from build123d import *

# Parameters (mm, degrees)
SKETCH1_W                      = 20
SKETCH1_H                      = 16
BOSS_EXTRUDE1_DEPTH            = 11.5
CUT_EXTRUDE1_DEPTH             = 17
SKETCH3_W                      = 3
SKETCH3_H                      = 16
SKETCH4_W                      = 1.5
SKETCH4_H                      = 7
F_6_0_6_DIAMETER_HOLE1_D       = 6
F_6_0_6_DIAMETER_HOLE1_DEPTH   = 11.5
F_3_0_3_DIAMETER_HOLE2_D       = 3
F_3_0_3_DIAMETER_HOLE2_DEPTH   = 3.5
F_3_0_3_DIAMETER_HOLE3_D       = 3
F_3_0_3_DIAMETER_HOLE3_DEPTH   = 3.5
F_1_5_1_5_DIAMETER_HOLE1_D     = 1.5
F_1_5_1_5_DIAMETER_HOLE1_DEPTH = 4.5
CHAMFER1_SIZE                  = 0.25


with BuildPart() as part:
    # Sketch1 → Boss-Extrude1 (new body)
    with BuildSketch(Plane.XZ):
        Rectangle(SKETCH1_W, SKETCH1_H)
    extrude(amount=-BOSS_EXTRUDE1_DEPTH)

    # Sketch2 → Cut-Extrude1 (cut, through all)
    with BuildSketch(Plane(origin=(0, 0, -8), x_dir=(-1, 0, 0), z_dir=(0, 0, -1))):
        with BuildLine():
            Line((10, 3.5), (10, 4.5))
            Line((10, 4.5), (4.458039892, 4.5))
            ThreePointArc((4.458039892, 4.5), (4.5, 4), (4.458039892, 3.5))
            Line((4.458039892, 3.5), (10, 3.5))
        make_face()
    extrude(amount=-CUT_EXTRUDE1_DEPTH, mode=Mode.SUBTRACT)

    # Sketch3 → Cut-Revolve1 (revolve, cut)
    with BuildSketch(Plane(origin=(0, 4, 0), x_dir=(1, 0, 0), z_dir=(0, 1, 0))):
        Rectangle(SKETCH3_W, SKETCH3_H)
    revolve(axis=Axis((-1.5, 4, -8), (0, 0, 1)), mode=Mode.SUBTRACT)

    # Sketch4 → Ø3.0 (3) Diameter Hole1 (revolve, cut)
    with BuildSketch(Plane(origin=(-7.5, 4.5, 0), x_dir=(0, 0, -1), z_dir=(1, 0, 0))):
        with Locations((0.75, 3.5)):
            Rectangle(SKETCH4_W, SKETCH4_H)
    revolve(axis=Axis((-7.5, -1.85, 0), (0, 1, 0)), mode=Mode.SUBTRACT)

    # Ø6.0 (6) Diameter Hole1
    with Locations(Plane(origin=(0, 0, 0), x_dir=(-1, 0, 0), z_dir=(0, -1, 0))):
        with Locations((-5.5, 0)):
            Hole(F_6_0_6_DIAMETER_HOLE1_D / 2, depth=F_6_0_6_DIAMETER_HOLE1_DEPTH)

    # Ø3.0 (3) Diameter Hole2
    with Locations(Plane(origin=(0, 3.5, 0), x_dir=(1, 0, 0), z_dir=(0, 1, 0))):
        with Locations((-7.5, 0)):
            Hole(F_3_0_3_DIAMETER_HOLE2_D / 2, depth=F_3_0_3_DIAMETER_HOLE2_DEPTH)

    # Ø3.0 (3) Diameter Hole3
    with Locations(Plane.XY.offset(8)):
        with Locations((6.5, 4.8)):
            Hole(F_3_0_3_DIAMETER_HOLE3_D / 2, depth=F_3_0_3_DIAMETER_HOLE3_DEPTH)

    # Ø1.5 (1.5) Diameter Hole1
    with Locations(Plane.XY.offset(8)):
        with Locations((8, 2)):
            Hole(F_1_5_1_5_DIAMETER_HOLE1_D / 2, depth=F_1_5_1_5_DIAMETER_HOLE1_DEPTH)

    # Chamfer1
    chamfer1_edges = [part.edges().sort_by_distance(p)[0] for p in [
        (0, 11.5, 8),
        (-10, 11.5, 0),
        (-10, 1.75, 8),
        (-10, 1.75, -8),
        (0, 11.5, -8),
        (-10, 0, 0),
        (0, 0, 8),
        (10, 0, 0),
        (0, 0, -8),
        (10, 11.5, 0),
        (-10, 8, -8),
        (-10, 8, 8),
        (10, 5.75, 8),
        (10, 5.75, -8),
    ]]
    chamfer(chamfer1_edges, length=CHAMFER1_SIZE)


solid = part.part
The listing builds one solid part. Answer for the finished solid, in the listing's coordinates (mm). A direction names the side the tool comes from. Give positions to 0.01 mm unless a question says otherwise; leave off trailing zeros. Order: outer loops, then holes, each group sorted by start corner. A loop starts at its lowest first (then second) coordinate and runs counter-clockwise, first axis right, second up. Notation, with made-up numbers: (-12, -35) - (38, -35) arc R22 cw to (38, -18) - close; hole circle Ø1 at (-34.75, -9). An arc over 180 degrees is marked (long way). Answer as CSV lines item,"result".
Q1. A cutting plane is placed at B-B, the plane y = 2. Determine the outline of the cut face in (x, z), and give its area (3 significant figures).
Answer key:
outline,"(-10, -7.75) - (-9.75, -8) - (-3.74, -8) - (-3.74, 8) - (-9.75, 8) - (-10, 7.75) - close; (0.74, -8) - (9.75, -8) - (10, -7.75) - (10, 7.75) - (9.75, 8) - (8.75, 8) - (8.75, 3.5) - (7.25, 3.5) - (7.25, 8) - (0.74, 8) - close; hole circle Ø3 at (-7.5, 0); hole circle Ø6 at (5.5, 0)"
area,"206 mm^2"
Q2. Determine the mould class of faces 4 (the face through (0, 0, 0)), 5 (the face through (-6, 2, 0)), 6 (the face through (0, 11.5, 0)), 7 (the face through (8, 2, 3.5)) for opening direction Y: pulls with the +Y half, pulls with the -Y half, needs draft (parallel to the pull), parting line crosses it, or undercut.
Answer key:
face 4,"pulls with the -Y half"
face 5,"needs draft"
face 6,"pulls with the +Y half"
face 7,"undercut"
Q3. A cutting plane is placed at D-D, the plane z = 0. Determine the outline of the cut face in (x, y).
Answer key:
outline,"(-10, 0.25) - (-9.75, 0) - (-9, 0) - (-9, 3.5) - (-10, 3.5) - close; (-10, 4.5) - (-9, 4.5) - (-9, 11.5) - (-9.75, 11.5) - (-10, 11.25) - close; (-6, 0) - (2.5, 0) - (2.5, 11.5) - (-6, 11.5) - (-6, 4.5) - (-4.46, 4.5) arc R3 cw (long way) to (-4.46, 3.5) - (-6, 3.5) - close; (8.5, 0) - (9.75, 0) - (10, 0.25) - (10, 11.25) - (9.75, 11.5) - (8.5, 11.5) - close"
Q4. This flat-tipped pin is pushed along its axis until it touches: pin 1 Ø1.5 at (x, y) = (6.5, 5.5) entering from +Z. Where does it stop, or does it pass through?
Answer key:
pin 1,"stops at z = 4.5"
Q5. Which of the six approach directions +Z, -Z, +X, -X, +Y, -Y give full straight-line access (tool end or side, diameter ignored) to faces 1 (the face through (-7, 3.5, -2)), 2 (the face through (7, 5, 4.5)), 3 (the face through (8.27, 5.83, 1.15))?
Answer key:
face 1,"+Z, -Z, -X"
face 2,"+Z"
face 3,"+Y, -Y"
Q6. A cutting plane is placed at C-C, the plane x = -7.5. Determine the outline of the cut face in (y, z), and give its area (3 significant figures).
Answer key:
outline,"(0, -7.75) - (0.25, -8) - (3.5, -8) - (3.5, -1.5) - (0, -1.5) - close; (0, 1.5) - (3.5, 1.5) - (3.5, 8) - (0.25, 8) - (0, 7.75) - close; (4.5, -8) - (11.25, -8) - (11.5, -7.75) - (11.5, -1.5) - (4.5, -1.5) - close; (4.5, 1.5) - (11.5, 1.5) - (11.5, 7.75) - (11.25, 8) - (4.5, 8) - close"
area,"136 mm^2"
Q7. A cutting plane is placed at A-A, the plane z = 6.25. Determine the outline of the cut face in (x, y), and give its area (3 significant figures).
Answer key:
outline,"(-10, 0.25) - (-9.75, 0) - (9.75, 0) - (10, 0.25) - (10, 11.25) - (9.75, 11.5) - (-9.75, 11.5) - (-10, 11.25) - (-10, 4.5) - (-4.46, 4.5) arc R3 cw (long way) to (-4.46, 3.5) - (-10, 3.5) - close; hole circle Ø3 at (6.5, 4.8); hole circle Ø1.5 at (8, 2)"
area,"187 mm^2"
Q8. Straight lines are drawn through the part: L1, parallel to Z at x = 5.5, y = 1.75; L2, parallel to Z at x = 5.5, y = 5; L3, parallel to Y at x = -5.25, z = -1. For each, find the intervals that lie inside material, in ascending order.
Answer key:
L1,"z = -8 to -3, 3 to 8"
L2,"z = -8 to -3, 3 to 4.5"
L3,"y = 0 to 3.5, 4.5 to 11.5"
